For this review, take the finished solid that the model builds, in its own axes (mm). Face numbers are marked on the shaded views. A direction names the side the tool comes from. Coordinates: 2 decimals unless noted, no trailing zeros. Loops run counter-clockwise (first coordinate to the right, second up) from the corner with the lowest first, then second, coordinate; pieces in that order, holes last. Notation, with made-up numbers: M -40,49.5 L -29,49.5 A17 ccw -29,82.5 Z; hole C -36.75,28.25 d8. An arc over 180 degrees is marked long. Answer as a JSON object with one key per item and string values. Group by question number.
Item 1: Add section C-C (x = -2.25). State the section outline as (y, z) points, then the cut area to 3 significant figures.
Item 2: Wall thickness on L1, parallel to X at y = -14.5, z = 21; L2, parallel to X at y = -1, z = 0; L3, parallel to Y at x = -4, z = 0: over which ranges is each line inside the solid? List them lowest first. Write a range as from..to.
Item 3: Add section B-B (x = 0.5). State the section outline as (y, z) points.
Item 4: Tool access review of the marked faces 1 and 2: name each direction out of +Z, -Z, +X, -X, +Y, -Y from which nothing blocks a thin tool from reaching the whole face with its end or side.
Item 5: Add section A-A (z = 0). Count the separate pieces of the cut face and the enclosed holes in it, then the cut area to 3 significant figures.
Item 6: Insertion check: pin 1 (2 mm diameter, centred on y = -25, z = -14.5, fed in from +X); pin 2 (5 mm diameter, centred on x = -1.54, z = 0, fed in from -Y); pin 3 (4 mm diameter, centred on x = -8, y = -22, fed in from +Z). Each pin has a flat end and moves straight along its axis. Give the tip position at first contact, or say it passes through.
from build123d import *

# Parameters (mm, degrees)
CUT_EXTRUDE3_DEPTH      = 2
CUT_EXTRUDE3_DEPTH_BACK = 8
SKETCH7_R               = 1.5


with BuildPart() as part:
    # Sketch1 → Revolve1 (revolve)
    with BuildSketch(Plane.XY, mode=Mode.PRIVATE) as revolve1_sk:
        with BuildLine():
            Line((-11.54268079, 15.022902393), (-10.04268079, 15.022902393))
            ThreePointArc((-10.04268079, 15.022902393), (-9.689127399, 14.876455783), (-9.54268079, 14.522902393))
            Line((-9.54268079, 14.522902393), (-9.54268079, 13.022902453))
            ThreePointArc((-9.54268079, 13.022902453), (-8.54268079, 12.022902453), (-7.54268079, 13.022902453))
            Line((-7.54268079, 13.022902453), (-7.54268079, 14.522902393))
            ThreePointArc((-7.54268079, 14.522902393), (-7.396234181, 14.876455783), (-7.04268079, 15.022902393))
            Line((-7.04268079, 15.022902393), (-5.54268079, 15.022902393))
            Line((-5.54268079, 15.022902393), (-5.54268079, 0.522902393))
            ThreePointArc((-5.54268079, 0.522902393), (-5.396234181, 0.169349002), (-5.04268079, 0.022902393))
            Line((-5.04268079, 0.022902393), (2.45731921, 0.022902393))
            Line((2.45731921, 0.022902393), (2.45731921, -5.477097607))
            Line((2.45731921, -5.477097607), (-11.54268079, -5.477097607))
            Line((-11.54268079, -5.477097607), (-11.54268079, 15.022902393))
        make_face()
    revolve(revolve1_sk.sketch.rotate(Axis((-11.54268079, -7.977097607, 0), (1, 0, 0)), 90), axis=Axis((-11.54268079, -7.977097607, 0), (1, 0, 0)))

    # Sketch7 → Cut-Extrude3 (cut, two sides: drawn at the far end of the back side and taken through both)
    with BuildSketch(Plane(origin=(0, 0, 0), x_dir=(1, 0, 0), z_dir=(0, 1, 0)).offset(-CUT_EXTRUDE3_DEPTH_BACK)):
        with Locations(Location((-1.54268079, 0, 0), (0, 0, 90))):
            Circle(SKETCH7_R)
    extrude(amount=CUT_EXTRUDE3_DEPTH + CUT_EXTRUDE3_DEPTH_BACK, mode=Mode.SUBTRACT)


solid = part.part
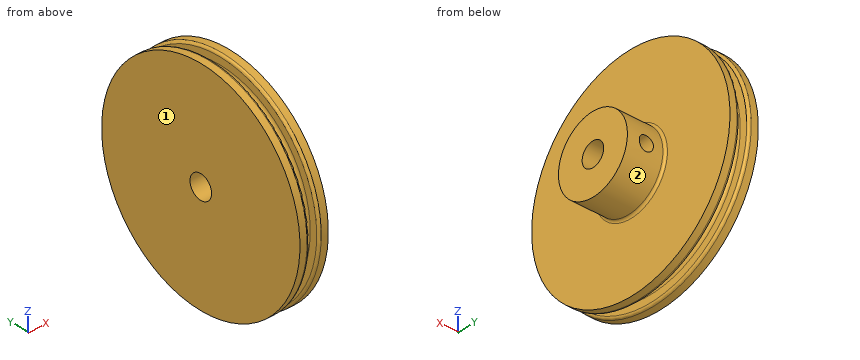
From the geometry:
{
 "1": {"outline": "M -5.86,-1.32 A2.5 cw long -5.86,1.32 L -0.09,1.32 A8 ccw long -0.09,-1.32 Z", "area": "167 mm²"},
 "2": {"L1": "x = -11.54..-9.54, -7.54..-5.54", "L2": "x = -11.54..-3.04, -0.04..2.46", "L3": "y = -15.98..-10.48, -5.48..0.02"},
 "3": {"outline": "C -7.98,0 d16; hole C -7.98,0 d5"},
 "4": {"face 1": "+Z, -Z, -X, +Y, -Y", "face 2": "+X"},
 "5": {"separate pieces": "3", "enclosed holes": "0", "area": "306 mm²"},
 "6": {"pin 1": "stops at x = -5.54", "pin 2": "stops at y = -15.98", "pin 3": "stops at z = 19.48"}
}
